from build123d import *

# Parameters (mm, degrees)
F_1_1_DIAMETER_HOLE1_D = 25.4
CIRPATTERN1_COUNT      = 5
FILLET2_R              = 10.795


with BuildPart() as part:
    # Sketch1 → Revolve1 (revolve)
    with BuildSketch(Plane.XY):
        Polygon((87.63, 0), (57.15, 0), (57.15, 10.795), (0, 10.795), (0, 20.955), (57.15, 20.955), (57.15, 31.75), (79.9973, 31.75), (79.9973, 28.0416), (87.63, 28.0416), align=None)
    revolve(axis=Axis((0, 10.795, 0), (0, 1, 0)))

    # 1 (1) Diameter Hole1 (through all)
    with Locations(Plane(origin=(0, 20.955, 0), x_dir=(1, 0, 0), z_dir=(0, 1, 0))):
        with Locations((0, 0)):
            Hole(F_1_1_DIAMETER_HOLE1_D / 2)

    # Sketch7 → 3/16 (0.187) Dowel Hole1 (revolve, cut)
    with BuildSketch(Plane(origin=(0, 31.75, -66.675), x_dir=(0, 0, 1), z_dir=(1, 0, 0))):
        Polygon((0, 0), (0, 11.078983884), (2.3749, 9.652), (2.3749, 0), align=None)
    f_3_16_0_187_dowel_hole1 = revolve(axis=Axis((0, 38.1, -66.675), (0, -1, 0)), mode=Mode.SUBTRACT)

    # CirPattern1: 3/16 (0.187) Dowel Hole1 ×5 about axis
    cirpattern1_axis = Axis((0, 0, 0), (0, 1, 0))
    for i in range(1, CIRPATTERN1_COUNT):
        add(f_3_16_0_187_dowel_hole1.rotate(cirpattern1_axis, i * 360 / CIRPATTERN1_COUNT), mode=Mode.SUBTRACT)

    # Fillet2
    fillet2_edges = [part.edges().sort_by_distance(p)[0] for p in [
        (-57.15, 10.795, 0),
        (-57.15, 20.955, 0),
    ]]
    fillet(fillet2_edges, radius=FILLET2_R - 0.0001)  # a hair under: the kernel refuses the full size


solid = part.part
For this review, take the finished solid that the model builds, in its own axes (mm). A direction names the side the tool comes from. Give positions to 0.01 mm unless a question says otherwise; leave off trailing zeros. Loops run counter-clockwise (first coordinate to the right, second up) from the corner with the lowest first, then second, coordinate; pieces in that order, holes last. Notation, with made-up numbers: M 68,21 L 87,21 A13 ccw 87,36 Z; hole C -34.75,33.25 d10. An arc over 180 degrees is marked long. Put each result on its own line as item: value. Start each with the question number.
(1) The part is to be moulded in two halves that separate along X. For faces 4 (the cylindrical face through (-65.572, 26.992, -19.618)), 5 (the cylindrical face through (-17.342, 29.87, 78.095)), 6 (the flat face through (-39, 28.042, 71)), 7 (the conical face through (63.34, 20.92, -21.01)), say which applies: +X half, -X half, draft (parallel to the pull), parting line (faces both ways), or undercut.
(2) For pin 1 (4.5 mm diameter, centred on x = -39.19, z = 53.94, fed in from +Y); pin 2 (5 mm diameter, centred on x = -62.5, z = -14.5, fed in from -Y); pin 3 (6 mm diameter, centred on x = -63.5, z = -67.5, fed in from +Y); pin 4 (6 mm diameter, centred on x = 26.5, y = 3.5, fed in from +Z), all flat-tipped, find the tip position at first contact; note any pin that passes through.
(3) Wall thickness on L1, parallel to Z at x = 0, y = 25; L2, parallel to Y at x = -1.5, z = 21.5 (3 decimals); L3, parallel to Z at x = 7.5, y = 17.5: over which ranges is each line inside the solid? List them lowest first.
(4) Add section B-B, the plane y = 25. Write out the cut boundary in (x, z) (3 decimals), then the cut area to 3 significant figures.
(5) Machinability: for faces 1 (the cylindrical face through (-0.71, 26.99, -64.41)), 2 (the flat face through (18.9, 31.75, -54.5)), 3 (the flat face through (10, 10.795, 10)), which of the approach directions +Z, -Z, +X, -X, +Y, -Y give a long, thin tool a straight path to every point of the face, cutting with its end or side? Answer none if there is none.
(6) Add section C-C, the plane y = 15. Write out the cut boundary in (x, z), then the cut area to 3 significant figures.
(7) Add section D-D, the plane z = 74. Write out the cut boundary in (x, y), then the cut area to 3 significant figures.
Result:
1. face 4: undercut
1. face 5: parting line
1. face 6: draft
1. face 7: undercut
2. pin 1: stops at y = 22.02
2. pin 2: stops at y = 0
2. pin 3: passes through
2. pin 4: stops at z = 84.42
3. L1: z = -87.63 to -69.05, -64.3 to -54.78, 54.78 to 87.63
3. L2: y = 10.795 to 20.955
3. L3: z = -87.31 to -10.25, 10.25 to 87.31
4. outline: C 0,0 d175.26; hole C -63.412,-20.604 d4.75; hole C 0,0 d109.559; hole C -39.191,53.941 d4.75; hole C 0,-66.675 d4.75; hole C 39.191,53.941 d4.75; hole C 63.412,-20.604 d4.75
4. area: 14,600 mm^2
5. face 1: +Y
5. face 2: +Z, -Z, +X, -X, +Y
5. face 3: -Y
6. outline: C 0,0 d175.26; hole C 0,0 d25.4
6. area: 23,600 mm^2
7. outline: M -46.94,0 L 46.94,0 L 46.94,28.04 L 30.39,28.04 L 30.39,31.75 L -30.39,31.75 L -30.39,28.04 L -46.94,28.04 Z
7. area: 2,860 mm^2
